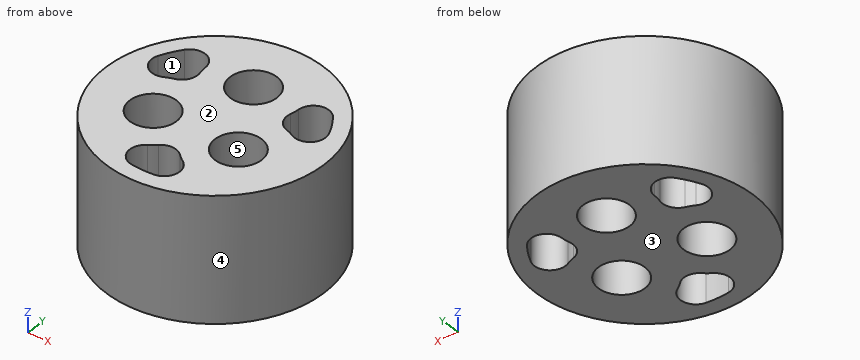
Autodesk Inventor part; units mm, degrees
ref_plane "YZ Plane" through (0, 0, 0) normal (1, 0, 0) x (0, 1, 0)
ref_plane "XZ Plane" through (0, 0, 0) normal (0, 1, 0) x (-1, 0, 0)
ref_plane "XY Plane" through (0, 0, 0) normal (0, 0, 1) x (1, 0, 0)
sketch "スケッチ1" plane through (0, 0, 0) normal (0, 0, 1) x (1, 0, 0)
  line L0 (0, 3.1754) -> (2.75, -1.5877)
  line L1 (2.75, -1.5877) -> (-2.75, -1.5877)
  line L2 (-2.75, -1.5877) -> (0, 3.1754)
  circle A0 centre (0, 3.1754) radius 1.5
  circle A1 centre (-2.75, -1.5877) radius 1.5
  circle A2 centre (2.75, -1.5877) radius 1.5
  circle A3 centre (0, 3.1754) radius 4
  circle A4 centre (-2.75, -1.5877) radius 4
  circle A5 centre (2.75, -1.5877) radius 4
  circle A6 centre (0, 0) radius 7.5
  circle A7 centre (0, 0) radius 4.6754
  circle A8 centre (0, 0) radius 7
  dimension "d0" = 3
  dimension "d1" = 3
  dimension "d2" = 3
  dimension "d3" = 2.5
  dimension "d4" = 2.5
  dimension "d5" = 2.5
  dimension "d6" = 15
  dimension "d7" = 2.8246
  dimension "d8" = 14
  dimension "d9" = 2.3246
extrude "押し出し1" add sketch "スケッチ1" against normal blind 8 contours A5 A3 L0 | A5 A4 A0 | A0 A7 A3 A5 | L0 A3 A4 A5 | A4 A5 A3 L2 | A4 A3 A7 A0 | L2 A3 A4 | A3 A5 A7 A2 | A2 A4 A3 | A3 A7 A5 | A4 A3 A5 | A3 A5 A1 | A1 A7 A4 A3 | A7 A3 A8 | A4 A7 A3 | A4 A5 L1 | L1 A5 A3 A4 | A2 A7 A5 A4 | A3 A8 A5 A7 | A5 A8 A7 | A5 A4 A7 A1 | A7 A4 A8 | A7 A4 A8 A3 | A5 A7 A4 | A7 A5 A8 A4
sketch "スケッチ2" plane through (0, 0, 0) normal (0, 0, 1) x (1, 0, 0)
  circle A0 centre (0, 0) radius 7
  circle A1 centre (2.75, -1.5877) radius 1.5
  circle A2 centre (-2.75, -1.5877) radius 1.5
  circle A3 centre (0, 3.1754) radius 1.5
  circle A4 centre (0, 3.1754) radius 4
  circle A5 centre (-2.75, -1.5877) radius 4
  circle A6 centre (2.75, -1.5877) radius 4
  circle A7 centre (0, 0) radius 4.5
  dimension "d12" = 2.5
  dimension "d13" = 2.5
  dimension "d14" = 2.5
  dimension "d15" = 2.5
sketch "スケッチ3" plane through (0, 0, 0) normal (0, 0, 1) x (1, 0, 0)
  circle A0 centre (0, 3.1754) radius 1.5
  circle A1 centre (-2.75, -1.5877) radius 1.5
  circle A2 centre (2.75, -1.5877) radius 1.5
  circle A3 centre (0, 0) radius 7
  circle A4 centre (0, 3.1754) radius 3
  circle A5 centre (-2.75, -1.5877) radius 3
  circle A6 centre (2.75, -1.5877) radius 3
  circle A7 centre (0, 0) radius 7
  circle A8 centre (0, 0) radius 6
  point P0 (-4.3667, -4.1148)
  point P1 (4.3667, -4.1148)
  point P2 (0, -2.7867)
  point P3 (5.7469, -1.7243)
  point P4 (1.3801, 5.8391)
  point P5 (2.4133, 1.3933)
  point P6 (-1.3801, 5.8391)
  point P7 (-5.7469, -1.7243)
  point P8 (-2.4133, 1.3933)
  dimension "d17" = 1
  dimension "d19" = 1.5
  dimension "d20" = 1.5
  dimension "d21" = 1.5
extrude "押し出し2" cut sketch "スケッチ3" against normal blind 10 contours A4 A8 A6 | A4 A5 A8 | A5 A6 A8
fillet "フィレット1" radius 1 9 edges at (-1.3801, 5.8391, -4) (1.3801, 5.8391, -4) (5.7469, -1.7243, -4) (2.4133, 1.3933, -4) (-2.4133, 1.3933, -4) (-5.7469, -1.7243, -4) (-4.3667, -4.1148, -4) (0, -2.7867, -4) (4.3667, -4.1148, -4)
equation "\"d3\" = d4"
equation "\"d5\" = d4"
equation "\"d20\" = d19"
equation "\"d21\" = d19"
properties part number "アーム 小さいカム" material "アルミニウム 2014-T6"
Verification items for the finished model (mm, model axes). Face numbers are marked on the shaded views. A direction names the side the tool comes from. Coordinates: 2 decimals unless noted, no trailing zeros. Write each loop counter-clockwise with the first axis right and the second up, starting at its lowest first coordinate (ties: lowest second). Pieces come first, ordered by that corner, then holes. Notation, with made-up numbers: (-16, -8.5) -> (1, -8.5) arc R21 ccw to (1, -4.5) -> close; hole circle Ø11 at (-18.5, 51). An arc over 180 degrees is marked (long way). One line per item, written item: value. Start each with the question number.
Q1. Thickness scan on L1, parallel to Y at x = 0, z = -3; L2, parallel to Y at x = -1, z = -3; L3, parallel to X at y = -2.25, z = -6. Record the ranges inside material, lowest first. Write a range as from..to.
Q2. Access from +Z, -Z, +X, -X, +Y, -Y to the whole of each face (thin tool, end or side, straight path). Record for the marked faces 1 and 2.
Q3. Cross-section at C-C on x = 2.25. Enter the section's corners in (y, z), and give its area (3 significant figures).
Q4. Go/stop test with flat-tipped pins: P1, Ø5, axis at x = 2.75, y = -1.59, coming from the +Z side; P2, Ø3, axis at y = -5, z = -3, coming from the +X side; P3, Ø1, axis at y = -5.5, z = -5.5, coming from the -X side; P4, Ø3, axis at y = 3, z = -3.5, coming from the +X side. Record where each tip stops, or that it passes through.
Q5. Cross-section at B-B on x = 0. State how many separate pieces and enclosed holes the cut face has, and give its area (3 significant figures).
Q6. Cross-section at D-D on y = -2.25. Enter the section's corners in (x, z), and give its area (3 significant figures).
Q7. Cross-section at A-A on y = 4.5. Enter the section's corners in (x, z), and give its area (3 significant figures).
Q8. Mould release check, pull along Y, two halves, no side actions. Record for the marked faces 3, 4 and 5: pulls with the +Y half, pulls with the -Y half, needs draft (parallel to the pull), parting line crosses it, or undercut.
Checked values:
1. L1: y = -7..-6, -3.49..1.68, 4.68..7
1. L2: y = -6.93..-5.88, -4.02..2.06, 4.29..6.93
1. L3: x = -6.63..-4.1, -1.4..1.4, 4.1..6.63
2. face 1: +Z, -Z
2. face 2: +Z, +X, -X, +Y, -Y
3. outline: (-6.63, -8) -> (-3, -8) -> (-3, 0) -> (-6.63, 0) -> close; (-0.17, -8) -> (6.63, -8) -> (6.63, 0) -> (-0.17, 0) -> close
3. area: 83.4 mm²
4. P1: stops at z = 0
4. P2: stops at x = 6.06
4. P3: stops at x = -4.9
4. P4: stops at x = 6.84
5. separate pieces: 3
5. enclosed holes: 0
5. area: 67.9 mm²
6. outline: (-6.63, -8) -> (-4.1, -8) -> (-4.1, 0) -> (-6.63, 0) -> close; (-1.4, -8) -> (1.4, -8) -> (1.4, 0) -> (-1.4, 0) -> close; (4.1, -8) -> (6.63, -8) -> (6.63, 0) -> (4.1, 0) -> close
6. area: 63.0 mm²
7. outline: (-5.36, -8) -> (-0.7, -8) -> (-0.7, 0) -> (-5.36, 0) -> close; (0.7, -8) -> (5.36, -8) -> (5.36, 0) -> (0.7, 0) -> close
7. area: 74.5 mm²
8. face 3: needs draft
8. face 4: parting line crosses it
8. face 5: undercut
